Check sheet for the modelled part. Datum: model origin and axes. Units: mm. Coordinates: 2 decimals unless noted, no trailing zeros. Loops run counter-clockwise (first coordinate to the right, second up) from the corner with the lowest first, then second, coordinate; pieces in that order, holes last. Notation, with made-up numbers: (89.5, 80.5) - (135.5, 80.5) arc R15 cw to (135.5, 104.5) - close; hole circle Ø1 at (-23, -33). An arc over 180 degrees is marked (long way). Answer as a JSON object with one key per item and string values. Group by question number.
from build123d import *

# Parameters (mm, degrees)
F0_W     = 5
F0_H     = 14
F0_W_2   = 108
F1_DEPTH = 0.35


with BuildPart() as f1:
    # F0 (on Top) → F1 (new body)
    with BuildSketch(Plane.XY):
        with BuildLine():
            ThreePointArc((54, 44.5), (52.5355339059, 48.0355339059), (49, 49.5))
            Line((49, 49.5), (-49, 49.5))
            ThreePointArc((-49, 49.5), (-52.5355339059, 48.0355339059), (-54, 44.5))
            Line((-54, 44.5), (-54, 32))
            Line((-54, 32), (54, 32))
            Line((54, 32), (54, 44.5))
        make_face()
        with Locations((56.5, 25)):
            Rectangle(F0_W, F0_H)
        Polygon((54, 18), (54, 32), (-54, 32), (-54, 18), (0, 18), align=None)
        with Locations((-56.5, 25)):
            Rectangle(F0_W, F0_H)
        Polygon((54, -18), (54, 18), (0, 18), (-54, 18), (-54, -18), align=None)
        with Locations((56.5, -25)):
            Rectangle(F0_W, F0_H)
        with Locations((0, -25)):
            Rectangle(F0_W_2, F0_H)
        with Locations((-56.5, -25)):
            Rectangle(F0_W, F0_H)
        with BuildLine():
            Line((54, -44.5), (54, -32))
            Line((54, -32), (-54, -32))
            Line((-54, -32), (-54, -44.5))
            ThreePointArc((-54, -44.5), (-52.5355339059, -48.0355339059), (-49, -49.5))
            Line((-49, -49.5), (49, -49.5))
            ThreePointArc((49, -49.5), (52.5355339059, -48.0355339059), (54, -44.5))
        make_face()
    extrude(amount=F1_DEPTH)


solid = f1.part
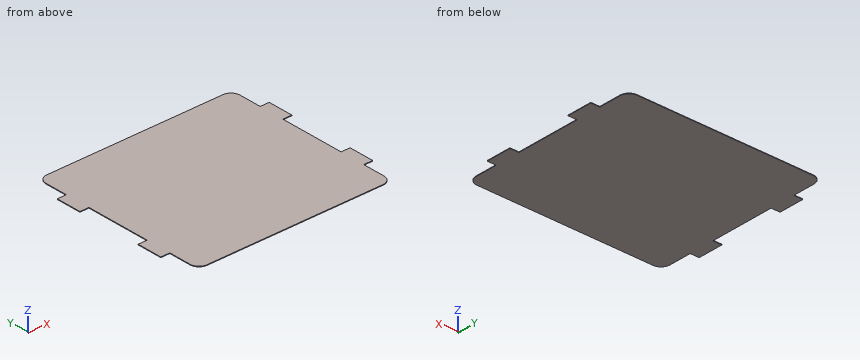
1. Sectioned sample at A-A on z = 0.1. Record the cut outline in (x, y), plus the area to 3 significant figures.
2. Sectioned sample at B-B on y = 9. Record the cut outline in (x, z).
3. Material ranges on line 1 (X direction, y = -7, z = 0.05); line 2 (Y direction, x = 53, z = 0.1), recorded low to high.
Answers follow:
{
 "1": {"outline": "(-59, -32) - (-54, -32) - (-54, -44.5) arc R5 ccw to (-49, -49.5) - (49, -49.5) arc R5 ccw to (54, -44.5) - (54, -32) - (59, -32) - (59, -18) - (54, -18) - (54, 18) - (59, 18) - (59, 32) - (54, 32) - (54, 44.5) arc R5 ccw to (49, 49.5) - (-49, 49.5) arc R5 ccw to (-54, 44.5) - (-54, 32) - (-59, 32) - (-59, 18) - (-54, 18) - (-54, -18) - (-59, -18) - close", "area": "11,000 mm^2"},
 "2": {"outline": "(-54, 0) - (54, 0) - (54, 0.35) - (-54, 0.35) - close"},
 "3": {"line 1": "x = -54 to 54", "line 2": "y = -47.5 to 47.5"}
}
